Could you check a few things on this drawing? It's one solid part, dimensions in mm from its lowest x, y, z. A direction names the side the tool comes from. Give positions to 0.01 mm unless a question says otherwise; leave off trailing zeros. Order: outer loops, then holes, each group sorted by start corner. A loop starts at its lowest first (then second) coordinate and runs counter-clockwise, first axis right, second up. Notation, with made-up numbers: M -11.75,-24.5 L 27.25,-24.5 A29 cw 27.25,7.5 Z; hole C 59,-22.5 d2. An arc over 180 degrees is marked long. Use one line per item in the form item = value.
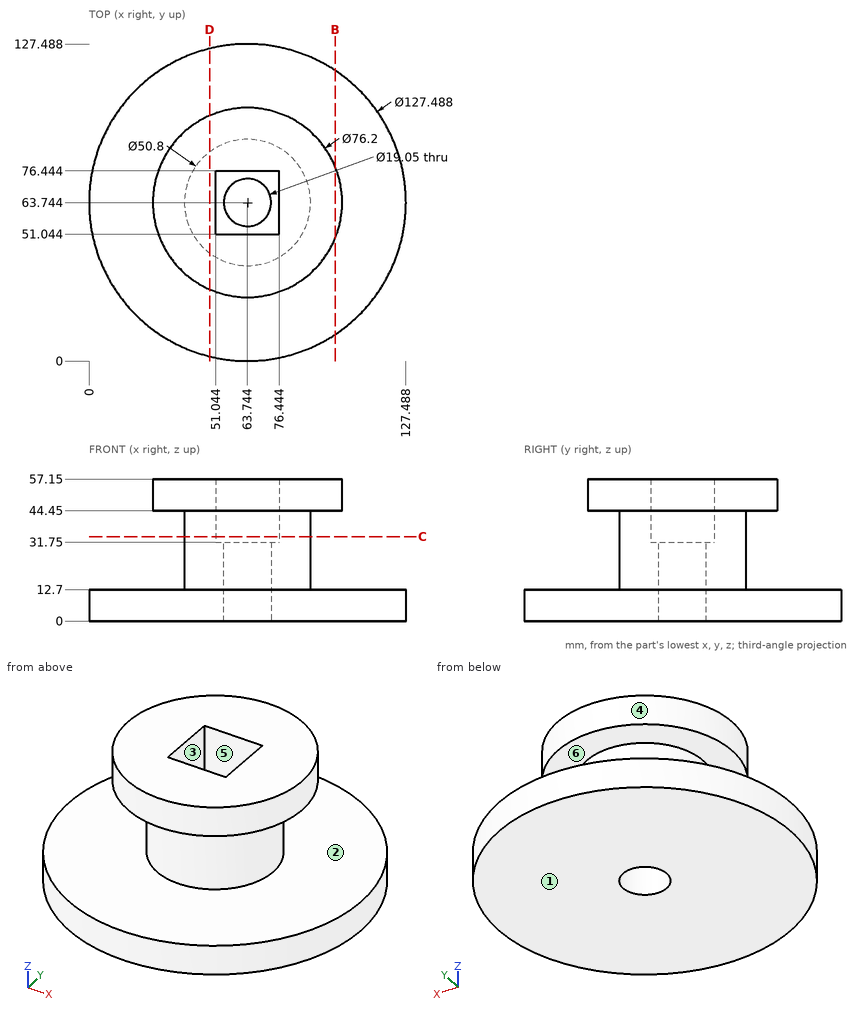
Q1. I need wall thicknesses on L1, parallel to Z at x = 89, y = 46; L2, parallel to Z at x = 11, y = 90.5; L3, parallel to X at y = 71, z = 33.5 (1 decimal). Which ranges of each line are inside material? Lowest first, please.
Found:
L1 = 0 to 12.7, 44.45 to 57.15
L2 = 0 to 12.7
L3 = 39.4 to 51, 76.4 to 88.1
Q2. Thinking about a two-plate mould opening in X: for the marked faces 3, 4, 5 and 6, which applies, +X half, -X half, draft (parallel to the pull), parting line (faces both ways), or undercut?
Found:
face_3 = undercut
face_4 = parting line
face_5 = undercut
face_6 = draft
Q3. I want a section at D-D on x = 48.5. Write out the boundary of the cut face in (y, z), then the cut area to 3 significant figures.
Found:
outline = M 1.85,0 L 125.64,0 L 125.64,12.7 L 84.06,12.7 L 84.06,44.45 L 98.66,44.45 L 98.66,57.15 L 28.83,57.15 L 28.83,44.45 L 43.43,44.45 L 43.43,12.7 L 1.85,12.7 Z
area = 3,750 mm²
Q4. On a 3-axis mill with a long thin cutter (end or side, diameter ignored), from which of +Z, -Z, +X, -X, +Y, -Y can I reach the whole of each face in a straight line? I mean the marked faces 1 and 2. Say none if no direction works.
Found:
face_1 = -Z, +X, -X, +Y, -Y
face_2 = none
Q5. I'm going to push flat-ended pins straight in: pin 1 Ø4 at (y, z) = (60, 35.5) entering from -X; pin 2 Ø12 at (x, z) = (67, 43.5) entering from -Y; pin 3 Ø12.5 at (y, z) = (63, 44.5) entering from +X; pin 4 Ø2 at (x, y) = (22, 55) entering from -Z. Where does each tip first touch, or does it pass through?
Found:
pin_1 = 38.4
pin_2 = 25.64
pin_3 = 101.84
pin_4 = 0
Q6. I want a section at C-C on z = 34. Write out the boundary of the cut face in (x, y) (1 decimal).
Found:
outline = C 63.7,63.7 d50.8; hole M 51,51 L 76.4,51 L 76.4,76.4 L 51,76.4 Z
Q7. I want a section at B-B on x = 99. Write out the boundary of the cut face in (y, z), then the cut area to 3 significant figures.
Found:
outline = M 10.64,0 L 116.85,0 L 116.85,12.7 L 10.64,12.7 Z; M 49.3,44.45 L 78.19,44.45 L 78.19,57.15 L 49.3,57.15 Z
area = 1,720 mm²
